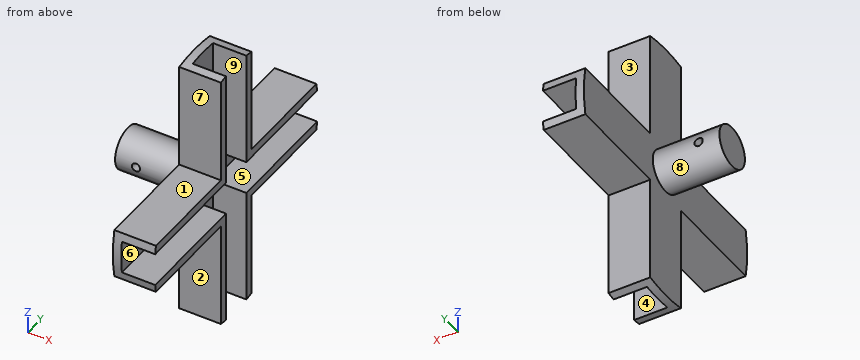
Autodesk Inventor part; units mm, degrees
ref_plane "YZ Plane" through (0, 0, 0) normal (1, 0, 0) x (0, 1, 0)
ref_plane "XZ Plane" through (0, 0, 0) normal (0, 1, 0) x (-1, 0, 0)
ref_plane "XY Plane" through (0, 0, 0) normal (0, 0, 1) x (1, 0, 0)
sketch "Sketch1" plane through (0, 0, 0) normal (1, 0, 0) x (0, 1, 0)
  circle A0 centre (0, 0) radius 32
  dimension "d0" = 64
extrude "Extrusion1" add sketch "Sketch1" along normal blind 10
sketch "Sketch2" plane through (10, 0, 0) normal (1, 0, 0) x (0, 0, -1)
  circle A0 centre (0, 0) radius 32
  line L0 (-6, 33.1057) -> (-6, 6)
  line L1 (-6, 6) -> (-33.1057, 6)
  line L2 (0, 0) -> (-11.4167, 0)
  line L3 (0, 0) -> (0, 10.4167)
  arc A1 (-6, 33.1057) -> (-33.1057, 6) centre (-1.4332, 1.4332) ccw
  line L4 (-6, -33.1057) -> (-6, -6)
  line L5 (-6, -6) -> (-33.1057, -6)
  arc A2 (-33.1057, -6) -> (-6, -33.1057) centre (-1.4332, -1.4332) ccw
  line L6 (6, 33.1057) -> (6, 6)
  line L7 (6, 6) -> (33.1057, 6)
  arc A3 (33.1057, 6) -> (6, 33.1057) centre (1.4332, 1.4332) ccw
  arc A4 (6, -33.1057) -> (33.1057, -6) centre (1.4332, -1.4332) ccw
  line L8 (6, -33.1057) -> (6, -6)
  line L9 (6, -6) -> (33.1057, -6)
  dimension "d3" = 12
  dimension "d4" = 12
extrude "Extrusion2" cut sketch "Sketch2" against normal blind 10 contours L7 L6 A0 | A0 L6 A3 L7 | L9 A4 L8 A0 | A0 L8 L9 | L0 L1 A0 | A0 L1 A1 L0 | L4 A2 L5 A0 | A0 L5 L4
shell "Shell1" thickness 2 removed faces 5 at (6.6667, 31.8245, -3.347) at (10, -0.6702, -14.6456) at (6.6667, 0.6706, -31.993) at (6.6667, -31.993, -0.6706) at (6.6667, -0.6706, 31.993)
sketch "Sketch3" plane through (0, 0, 0) normal (-1, 0, 0) x (0, 0, 1)
  arc A0 (-31.4325, 6) -> (-31.4325, -6) centre (0, 0) ccw
  circle A1 centre (0, 0) radius 5
  dimension "d9" = 10
extrude "Extrusion3" add sketch "Sketch3" along normal blind 16
sketch "Sketch4" plane through (0, 0, 0) normal (0, 1, 0) x (-1, 0, 0)
  circle A0 centre (11, 0) radius 1
  line L0 (16, -5) -> (16, 5)
  point P0 (0, 0)
  dimension "d12" = 2
  dimension "d13" = 5
extrude "Extrusion4" cut sketch "Sketch4" along normal mid plane 16
properties part number "Cross"
Could you check a few things on this model? Use its own coordinates, in mm. Face numbers are marked on the shaded views. A direction names the side the tool comes from. Round coordinates to 2 decimals unless told otherwise and drop trailing zeros. Loops run counter-clockwise (first coordinate to the right, second up) from the corner with the lowest first, then second, coordinate; pieces in that order, holes last. Notation, with made-up numbers: M 50.25,65.5 L 81.25,65.5 A15 cw 81.25,83.5 Z; hole C 64,11 d6. An arc over 180 degrees is marked long. Put each result on its own line as item: value.
Q1. Imagine slicing it at B-B (z = 0). Write out the boundary of the cut face in (x, y).
Check result:
outline: M -16,-5 L -12,-5 L -12,5 L -16,5 Z; M -10,-5 L 0,-5 L 0,-32 L 2,-32 L 2,32 L 0,32 L 0,5 L -10,5 Z
Q2. Imagine slicing it at D-D (z = 21). Write out the boundary of the cut face in (x, y).
Check result:
outline: M 0,-6 L 10,-6 L 10,-4 L 2,-4 L 2,4 L 10,4 L 10,6 L 0,6 Z
Q3. Imagine slicing it at A-A (y = 0). Write out the boundary of the cut face in (x, z), then the cut area to 3 significant figures.
Check result:
outline: M -16,-5 L 0,-5 L 0,-32 L 2,-32 L 2,32 L 0,32 L 0,5 L -16,5 Z; hole C -11,0 d2
area: 285 mm2
Q4. I need wall thicknesses on probe 1 along X at (y, z) = (0, 0); probe 2 along Y at (x, z) = (2.5, 22). Which ranges of each line are inside material? Lowest first, please.
Check result:
probe 1: -16 to -12, -10 to 2
probe 2: -6 to -4, 4 to 6
Q5. For pin 1 (11 mm diameter, centred on x = 4, z = -13, fed in from -Y); pin 2 (8 mm diameter, centred on x = 0.5, z = -18, fed in from +Y); pin 3 (2.5 mm diameter, centred on x = 5, y = 14, fed in from -Z), each with a flat end and sliding along its axis, tell me the tip position at first contact or that it passes through.
Check result:
pin 1: y = -6
pin 2: y = 6
pin 3: z = -6
Q6. Imagine slicing it at C-C (x = 8.5). Write out the boundary of the cut face in (y, z), then the cut area to 3 significant figures.
Check result:
outline: M -31.75,-4 A32 ccw -31.43,-6 L -6,-6 L -6,-31.43 A32 ccw -4,-31.75 L -4,-4 Z; M -31.75,4 L -4,4 L -4,31.75 A32 ccw -6,31.43 L -6,6 L -31.43,6 A32 ccw Z; M 4,-31.75 A32 ccw 6,-31.43 L 6,-6 L 31.43,-6 A32 ccw 31.75,-4 L 4,-4 Z; M 4,4 L 31.75,4 A32 ccw 31.43,6 L 6,6 L 6,31.43 A32 ccw 4,31.75 Z
area: 426 mm2
Q7. On a 3-axis mill with a long thin cutter (end or side, diameter ignored), from which of +Z, -Z, +X, -X, +Y, -Y can I reach the whole of each face in a straight line? I mean the marked faces 1, 2, 3, 4 and 5. Say none if no direction works.
Check result:
face 1: +Z, +X, -X, -Y
face 2: -Z, +X, -X, -Y
face 3: +Z, +X, -X, +Y
face 4: +Z, -Z, +X
face 5: +X, +Y, -Y
Q8. Thinking about a two-plate mould opening in Y: for the marked faces 6, 7, 8 and 9, which applies, released by +Y, released by -Y, zero draft, split by the parting line, or undercut?
Check result:
face 6: undercut
face 7: released by -Y
face 8: split by the parting line
face 9: undercut
